Model file for the job. Use its own axes, mm. A direction names the side the tool comes from. Coordinates: 2 decimals unless noted, no trailing zeros. Order: outer loops, then holes, each group sorted by start corner. A loop starts at its lowest first (then second) coordinate and runs counter-clockwise, first axis right, second up. Notation, with made-up numbers: M 54.5,44 L 103.5,44 A6 ccw 103.5,49 Z; hole C 69,66 d9. An arc over 180 degrees is marked long. Return JSON: item names as keys, results as strings.
```python
from build123d import *

# Parameters (mm, degrees)
SKETCH_1_W          = 60
SKETCH_1_H          = 70
SKETCH_1_R          = 2.5
EXTRUDE_1_DEPTH     = 1.8
SKETCH_2_R          = 1.5
SKETCH_2_W          = 40
SKETCH_2_H          = 36
CUT_EXTRUDE_1_DEPTH = 47.132851635
FILLET_1_R          = 2


with BuildPart() as part:
    # 草图1 → 凸台-拉伸1 (new body)
    with BuildSketch(Plane(origin=(0, 0, 0), x_dir=(1, 0, 0), z_dir=(0, 1, 0))):
        Rectangle(SKETCH_1_W, SKETCH_1_H)
        with Locations(Location((-20, 23, 0), (0, 0, 270))):
            Circle(SKETCH_1_R, mode=Mode.SUBTRACT)
        with Locations(Location((20, 23, 0), (0, 0, 90))):
            Circle(SKETCH_1_R, mode=Mode.SUBTRACT)
        with Locations(Location((20, -23, 0), (0, 0, 270))):
            Circle(SKETCH_1_R, mode=Mode.SUBTRACT)
        with Locations(Location((-20, -23, 0), (0, 0, 90))):
            Circle(SKETCH_1_R, mode=Mode.SUBTRACT)
    extrude(amount=EXTRUDE_1_DEPTH)

    # 草图2 → 切除-拉伸1 (cut, through all)
    with BuildSketch(Plane(origin=(0, 1.8, 0), x_dir=(1, 0, 0), z_dir=(0, 1, 0))):
        with Locations(Location((-25, 30, 0), (0, 0, 270))):
            Circle(SKETCH_2_R)
        with Locations(Location((25, 30, 0), (0, 0, 90))):
            Circle(SKETCH_2_R)
        with Locations(Location((25, -30, 0), (0, 0, 270))):
            Circle(SKETCH_2_R)
        with Locations(Location((-25, -30, 0), (0, 0, 90))):
            Circle(SKETCH_2_R)
        Rectangle(SKETCH_2_W, SKETCH_2_H)
    extrude(amount=-CUT_EXTRUDE_1_DEPTH, mode=Mode.SUBTRACT)

    # 圆角1
    fillet_1_edges = [part.edges().sort_by_distance(p)[0] for p in [
        (20, 0.9, -18),
        (20, 0.9, 18),
        (-20, 0.9, 18),
        (-20, 0.9, -18),
        (30, 0.9, 35),
        (-30, 0.9, 35),
        (-30, 0.9, -35),
        (30, 0.9, -35),
    ]]
    fillet(fillet_1_edges, radius=FILLET_1_R)


solid = part.part
```
Item 1: Saw through at D-D (x = 25). Write the cut outline in (y, z), and give its area (3 significant figures).
Check result:
{"outline": "M 0,-35 L 1.8,-35 L 1.8,-31.5 L 0,-31.5 Z; M 0,-28.5 L 1.8,-28.5 L 1.8,28.5 L 0,28.5 Z; M 0,31.5 L 1.8,31.5 L 1.8,35 L 0,35 Z", "area": "115 mm2"}
Item 2: Drop a flat-ended pin along its axis: pin 1 Ø4 at (x, z) = (20, 23) entering from -Y. Give the stop position or say it passes through.
Check result:
{"pin 1": "passes through"}
Item 3: 3-axis set-ups, long thin cutter, end or side, ignore diameter. For faces 4 (the flat face through (-20, 1, 0)), 5 (the cylindrical face through (29.4, 0.91, -34.43)): which of +Z, -Z, +X, -X, +Y, -Y reach the whole face in a straight line?
Check result:
{"face 4": "+Y, -Y", "face 5": "-Z, +X, +Y, -Y"}
Item 4: Wall check: line 1 (X direction, y = 1.35, z = -30); line 2 (Z direction, x = 1.5, y = 1.4); line 3 (X direction, y = 0.1, z = 10). Give the ranges that are in metal, low to high.
Check result:
{"line 1": "x = -30 to -26.5, -23.5 to 23.5, 26.5 to 30", "line 2": "z = -35 to -18, 18 to 35", "line 3": "x = -30 to -20, 20 to 30"}
Item 5: Saw through at A-A (z = 23). Write the cut outline in (x, y).
Check result:
{"outline": "M -30,0 L -22.5,0 L -22.5,1.8 L -30,1.8 Z; M -17.5,0 L 17.5,0 L 17.5,1.8 L -17.5,1.8 Z; M 22.5,0 L 30,0 L 30,1.8 L 22.5,1.8 Z"}
Item 6: Pull direction Z, two halves, no side cores. Call faces 1 (the cylindrical face through (-19.4, 0.89, 17.43)), 2 (the flat face through (-20.4, 0, -0.5)), 3 (the cylindrical face through (29.4, 0.91, 34.43)): +Z half, -Z half, draft (parallel to the pull), parting line (faces both ways), or undercut.
Check result:
{"face 1": "undercut", "face 2": "draft", "face 3": "+Z half"}
Item 7: Saw through at B-B (x = 15.5). Write the cut outline in (y, z).
Check result:
{"outline": "M 0,-35 L 1.8,-35 L 1.8,-18 L 0,-18 Z; M 0,18 L 1.8,18 L 1.8,35 L 0,35 Z"}
Item 8: Saw through at C-C (y = 0.7). Count the separate pieces of the cut face and the enclosed holes in it, and give its area (3 significant figures).
Check result:
{"separate pieces": "1", "enclosed holes": "9", "area": "2,650 mm2"}
